Check sheet for the modelled part. Datum: model origin and axes. Units: mm. A direction names the side the tool comes from. Round coordinates to 2 decimals unless told otherwise and drop trailing zeros. Order: outer loops, then holes, each group sorted by start corner. A loop starts at its lowest first (then second) coordinate and runs counter-clockwise, first axis right, second up.
(1) Depth check by flat-ended pin: pin 1 (4 mm diameter, centred on x = -11, z = -10.5, fed in from +Y); pin 2 (8 mm diameter, centred on y = 15.5, z = -7, fed in from +X). Enter the tip coordinate at first touch or a pass-through.
(2) Sectioned sample at B-B, the plane z = 6. Enter the section's corners in (x, y).
(3) Sectioned sample at D-D, the plane x = -10. Enter the section's corners in (y, z), and give its area (3 significant figures).
(4) Sectioned sample at C-C, the plane x = 1. Enter the section's corners in (y, z), and give its area (3 significant figures).
(5) Mould release check, pull along X, two halves, no side actions. Record for faces 1 (the flat face through (-7.5, 1, -14)), 2 (the cylindrical face through (-17.4, 10.85, 17.43)), 3 (the flat face through (16.4, 22, 16.4)): released by +X, released by -X, zero draft, split by the parting line, or undercut.
(6) Sectioned sample at A-A, the plane y = 4.75. Enter the section's corners in (x, z).
(7) Tool access check on faces 4 (the cylindrical face through (-17.43, 10.85, -17.4)), 5 (the cylindrical face through (13.242, 12.874, 13.371)), 6 (the flat face through (-14, 1, 7.5)). Record the directions out of +Z, -Z, +X, -X, +Y, -Y that give a thin tool (end or side, any length) a straight path to the whole face; none if there is none.
(8) Thickness scan on probe 1 along Z at (x, y) = (15.25, 8); probe 2 along X at (y, z) = (2.5, 14.5). Record the ranges inside material, lowest first.
Autodesk Inventor part; units mm, degrees
ref_plane "YZ Plane" through (0, 0, 0) normal (1, 0, 0) x (0, 1, 0)
ref_plane "XZ Plane" through (0, 0, 0) normal (0, 1, 0) x (-1, 0, 0)
ref_plane "XY Plane" through (0, 0, 0) normal (0, 0, 1) x (1, 0, 0)
sketch "Sketch1" plane through (0, 0, 0) normal (0, 1, 0) x (-1, 0, 0)
  line L0 (16, -18) -> (-16, -18)
  line L1 (-18, -16) -> (-18, 16)
  line L2 (-16, 18) -> (16, 18)
  line L3 (18, 16) -> (18, -16)
  line L4 (18, -18) -> (-18, 18)
  circle A0 centre (-15.25, -15.25) radius 1.35
  line L5 (0, -18) -> (0, 18)
  line L6 (18, 0) -> (-18, 0)
  circle A1 centre (-15.25, 15.25) radius 1.35
  circle A2 centre (15.25, -15.25) radius 1.35
  circle A3 centre (15.25, 15.25) radius 1.35
  arc A4 (16, -18) -> (18, -16) centre (16, -16) ccw
  arc A5 (-18, -16) -> (-16, -18) centre (-16, -16) ccw
  arc A6 (-16, 18) -> (-18, 16) centre (-16, 16) ccw
  arc A7 (18, 16) -> (16, 18) centre (16, 16) ccw
  point P0 (0, 0)
  point P1 (-18, -18)
  point P2 (18, 18)
  point P3 (0, 0)
  dimension "d0" = 36
  dimension "d1" = 36
  dimension "d4" = 2.7
  dimension "d5" = 30.5
  dimension "d6" = 30.5
  dimension "d7" = 2
extrude "Extrusion1" add sketch "Sketch1" along normal blind 2 contours L0 L5 L4 A2 A4 | L0 A5 L1 L6 L5 | L4 A2 L6 L3 A4 | L6 L1 A6 L4 A1 | L4 A1 A6 L2 L5 | L5 L2 A7 L3 L6
sketch "Sketch2" plane through (0, 2, 0) normal (0, 1, 0) x (1, 0, 0)
  circle A0 centre (-15.25, 15.25) radius 1.35
  circle A1 centre (15.25, 15.25) radius 1.35
  circle A2 centre (-15.25, -15.25) radius 1.35
  circle A3 centre (15.25, -15.25) radius 1.35
  circle A4 centre (-15.25, 15.25) radius 2.75
  line L0 (16, 18) -> (-16, 18)
  line L1 (0, 18) -> (0, -18)
  line L2 (-16, -18) -> (16, -18)
  line L3 (18, -16) -> (18, 16)
  line L4 (18, 0) -> (-18, 0)
  line L5 (-18, 16) -> (-18, -16)
  arc A5 (-16, 18) -> (-18, 16) centre (-16, 16) ccw
  line L6 (-16, -18) -> (16, -18)
  arc A6 (16, -18) -> (18, -16) centre (16, -16) ccw
  line L7 (18, -16) -> (18, 16)
  arc A7 (18, 16) -> (16, 18) centre (16, 16) ccw
  line L8 (16, 18) -> (-16, 18)
  arc A8 (-16, 18) -> (-18, 16) centre (-16, 16) ccw
  line L9 (-18, 16) -> (-18, -16)
  arc A9 (-18, -16) -> (-16, -18) centre (-16, -16) ccw
  circle A10 centre (15.25, 15.25) radius 1.35
  circle A11 centre (-15.25, 15.25) radius 1.35
  circle A12 centre (-15.25, -15.25) radius 1.35
  circle A13 centre (15.25, -15.25) radius 1.35
  circle A14 centre (15.25, 15.25) radius 2.75
  circle A15 centre (-15.25, -15.25) radius 2.75
  circle A16 centre (15.25, -15.25) radius 2.75
  point P0 (0, 0)
  point P1 (18, -15.25)
  point P2 (15.25, -18)
  point P3 (-15.25, -18)
  point P4 (-18, -15.25)
  point P5 (-18, -16)
  point P6 (15.25, 18)
  point P7 (18, 15.25)
  point P8 (-15.25, 18)
  point P9 (-18, 15.25)
extrude "Extrusion2" add sketch "Sketch2" along normal blind 20 contours A4 | A4 L5 A5 L0 | L0 A7 L3 A14 | A14 | A15 L2 A9 L5 | A15 | A16 L3 A6 L2 | A16
fillet "Fillet1" radius 2 4 edges at (-13.3055, 2, 13.3055) (13.3055, 2, 13.3055) (13.3055, 2, -13.3055) (-13.3055, 2, -13.3055)
sketch "Sketch3" plane through (0, 0, 0) normal (0, -1, 0) x (1, 0, 0)
  line L0 (-7.5, 16) -> (7.5, 16)
  line L1 (7.5, 16) -> (7.5, 12)
  line L2 (7.5, 12) -> (-7.5, 12)
  line L3 (-7.5, 12) -> (-7.5, 16)
  line L4 (-7.5, 12) -> (7.5, 16)
  line L5 (-16, 18) -> (16, 18)
  line L6 (0, 18) -> (0, -18)
  line L7 (11.377, -18) -> (-11.377, -18)
  line L8 (16, 7.5) -> (16, -7.5)
  line L9 (12, 7.5) -> (16, 7.5)
  line L10 (12, -7.5) -> (12, 7.5)
  line L11 (16, -7.5) -> (12, -7.5)
  line L12 (7.5, -16) -> (-7.5, -16)
  line L13 (7.5, -12) -> (7.5, -16)
  line L14 (-7.5, -12) -> (7.5, -12)
  line L15 (-7.5, -16) -> (-7.5, -12)
  line L16 (-16, -7.5) -> (-16, 7.5)
  line L17 (-12, -7.5) -> (-16, -7.5)
  line L18 (-12, 7.5) -> (-12, -7.5)
  line L19 (-16, 7.5) -> (-12, 7.5)
  point P0 (0, 0)
  point P1 (0, 14)
  point P2 (0, -12)
  point P3 (0, -16)
  dimension "d11" = 4
  dimension "d12" = 4
  dimension "d13" = 15
  dimension "d16" = 360
extrude "Extrusion3" cut sketch "Sketch3" against normal through all
properties part number "v3_gps_stand"
Derived:
1. pin 1: stops at y = 2.04
1. pin 2: passes through
2. outline: (-18, 0) - (-16, 0) - (-16, 2) - (-18, 2) - close; (-12, 0) - (12, 0) - (12, 2) - (-12, 2) - close; (16, 0) - (18, 0) - (18, 2) - (16, 2) - close
3. outline: (0, -18) - (2, -18) - (2, 18) - (0, 18) - close
3. area: 72.0 mm2
4. outline: (0, -18) - (2, -18) - (2, -16) - (0, -16) - close; (0, -12) - (2, -12) - (2, 12) - (0, 12) - close; (0, 16) - (2, 16) - (2, 18) - (0, 18) - close
4. area: 56.0 mm2
5. face 1: undercut
5. face 2: released by -X
5. face 3: zero draft
6. outline: (-18, -16) arc R2 ccw to (-16, -18) - (-15.25, -18) arc R2.75 ccw (long way) to (-18, -15.25) - close; (-18, 15.25) arc R2.75 ccw (long way) to (-15.25, 18) - (-16, 18) arc R2 ccw to (-18, 16) - close; (15.25, -18) - (16, -18) arc R2 ccw to (18, -16) - (18, -15.25) arc R2.75 ccw (long way) to start; (15.25, 18) arc R2.75 ccw (long way) to (18, 15.25) - (18, 16) arc R2 ccw to (16, 18) - close; hole circle Ø2.7 at (-15.25, -15.25); hole circle Ø2.7 at (-15.25, 15.25); hole circle Ø2.7 at (15.25, -15.25); hole circle Ø2.7 at (15.25, 15.25)
7. face 4: -Z, -X, +Y, -Y
7. face 5: +Y
7. face 6: +Y, -Y
8. probe 1: z = -18 to -16.6, -13.9 to -12.5, 12.5 to 13.9, 16.6 to 18
8. probe 2: x = -18 to -16.37, -14.13 to -11.91, 11.91 to 14.13, 16.37 to 18
